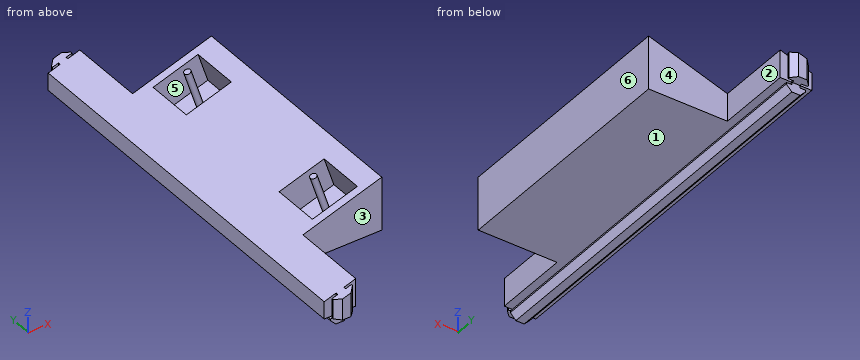
```python
from build123d import *

# Parameters (mm, degrees)
ESQUISSE1_W                   = 70
ESQUISSE1_H                   = 261.4
BOSS_EXTRU_1_DEPTH            = 40
ENL_V_MAT_EXTRU_1_DEPTH       = 335.841640665
ENL_V_MAT_EXTRU_1_DEPTH_BACK  = 40
ENL_V_MAT_EXTRU_2_DEPTH       = 335.841640665
ENL_V_MAT_EXTRU_2_DEPTH_BACK  = 40
ENL_V_MAT_EXTRU_3_DEPTH       = 287.347052656
ENL_V_MAT_EXTRU_3_DEPTH_BACK  = 165
ENL_V_MAT_EXTRU_4_DEPTH       = 328.480443637
ENL_V_MAT_EXTRU_4_DEPTH_BACK  = 261.4
ENL_V_MAT_EXTRU_5_DEPTH       = 328.480443637
ENL_V_MAT_EXTRU_5_DEPTH_BACK  = 261.4
ENL_V_MAT_EXTRU_6_DEPTH       = 335.841640665
ENL_V_MAT_EXTRU_6_DEPTH_BACK  = 40
ENL_V_MAT_EXTRU_8_DEPTH       = 335.841640665
ENL_V_MAT_EXTRU_8_DEPTH_BACK  = 40
ENL_V_MAT_EXTRU_9_DEPTH       = 281.544908808
ENL_V_MAT_EXTRU_9_DEPTH_BACK  = 40
ENL_V_MAT_EXTRU_10_DEPTH      = 335.841640665
ENL_V_MAT_EXTRU_10_DEPTH_BACK = 40
ENL_V_MAT_EXTRU_12_DEPTH      = 335.841640665
ENL_V_MAT_EXTRU_12_DEPTH_BACK = 40
ENL_V_MAT_EXTRU_14_DEPTH      = 280.494983601
ENL_V_MAT_EXTRU_14_DEPTH_BACK = 4.9
ENL_V_MAT_EXTRU_30_DEPTH      = 323.553128903
ENL_V_MAT_EXTRU_30_DEPTH_BACK = 323.553128903
ESQUISSE33_W                  = 30
ESQUISSE33_H                  = 30
ENL_V_MAT_EXTRU_34_DEPTH      = 20
ESQUISSE36_W                  = 30
ESQUISSE36_H                  = 30
ENL_V_MAT_EXTRU_35_DEPTH      = 20
ESQUISSE38_R                  = 2
BOSS_EXTRU_2_DEPTH            = 30
ESQUISSE39_R                  = 2
BOSS_EXTRU_3_DEPTH            = 30


with BuildPart() as part:
    # Esquisse1 → Boss.-Extru.1 (new body)
    with BuildSketch(Plane.XY):
        with Locations((-158.166976901, -139.865044598)):
            Rectangle(ESQUISSE1_W, ESQUISSE1_H)
    extrude(amount=BOSS_EXTRU_1_DEPTH)

    # Esquisse3 → Enlèv. mat.-Extru.1 (cut, two sides: drawn at the far end of the back side and taken through both)
    with BuildSketch(Plane.XY.offset(40).offset(-ENL_V_MAT_EXTRU_1_DEPTH_BACK)):
        Polygon((-173.166976901, 533.112927894), (-173.166976901, -9.165044598), (-173.166976901, -63.005044598), (-123.166976901, -63.005044598), (419.110995591, -63.005044598), (1188.481875045, 701.409795425), (596.203902553, 1297.527767917), align=None)
    extrude(amount=ENL_V_MAT_EXTRU_1_DEPTH + ENL_V_MAT_EXTRU_1_DEPTH_BACK, mode=Mode.SUBTRACT)

    # Esquisse4 → Enlèv. mat.-Extru.2 (cut, two sides: drawn at the far end of the back side and taken through both)
    with BuildSketch(Plane.XY.offset(40).offset(-ENL_V_MAT_EXTRU_2_DEPTH_BACK)):
        Polygon((-173.166976901, -812.84301709), (-173.166976901, -270.565044598), (-173.166976901, -216.725044598), (-123.166976901, -216.725044598), (419.110995591, -216.725044598), (1188.481875045, -981.139884621), (596.203902553, -1577.257857113), align=None)
    extrude(amount=ENL_V_MAT_EXTRU_2_DEPTH + ENL_V_MAT_EXTRU_2_DEPTH_BACK, mode=Mode.SUBTRACT)

    # Esquisse6 → Enlèv. mat.-Extru.3 (cut, two sides: drawn at the far end of the back side and taken through both)
    with BuildSketch(Plane(origin=(0, -63.005044598, 0), x_dir=(1, 0, 0), z_dir=(0, 1, 0)).offset(-ENL_V_MAT_EXTRU_3_DEPTH_BACK)):
        Polygon((42.299289537, -6.2), (-123.166976901, -6.2), (-173.166976901, -6.2), (-173.166976901, 0), (-173.166976901, 165.466266437), (33.046852916, 424.294776666), (248.513119354, 252.628510228), align=None)
    extrude(amount=ENL_V_MAT_EXTRU_3_DEPTH + ENL_V_MAT_EXTRU_3_DEPTH_BACK, mode=Mode.SUBTRACT)

    # Esquisse7 → Enlèv. mat.-Extru.4 (cut, two sides: drawn at the far end of the back side and taken through both)
    with BuildSketch(Plane(origin=(0, -9.165044598, 0), x_dir=(1, 0, 0), z_dir=(0, 1, 0)).offset(-ENL_V_MAT_EXTRU_4_DEPTH_BACK)):
        Polygon((-23.31660268, -6.2), (-173.166976901, -6.2), (-180.716976901, -6.2), (-180.716976901, -4.65), (-177.016976901, -4.65), (-177.016976901, -3.65), (-180.521416942, 0), (-284.304352032, 108.093649388), (-164.080204276, 382.623598415), (96.907545076, 268.329949026), align=None)
    extrude(amount=ENL_V_MAT_EXTRU_4_DEPTH + ENL_V_MAT_EXTRU_4_DEPTH_BACK, mode=Mode.SUBTRACT)

    # Esquisse8 → Enlèv. mat.-Extru.5 (cut, two sides: drawn at the far end of the back side and taken through both)
    with BuildSketch(Plane(origin=(0, -9.165044598, 0), x_dir=(1, 0, 0), z_dir=(0, 1, 0)).offset(-ENL_V_MAT_EXTRU_5_DEPTH_BACK)):
        Polygon((-358.633243338, -6.2), (-193.166976901, -6.2), (-185.616976901, -6.2), (-185.616976901, -4.65), (-189.316976901, -4.65), (-189.316976901, -3.65), (-185.81253686, 0), (-71.214392687, 119.358077569), (-203.692164198, 422.617012095), (-491.11101485, 297.058934527), align=None)
    extrude(amount=ENL_V_MAT_EXTRU_5_DEPTH + ENL_V_MAT_EXTRU_5_DEPTH_BACK, mode=Mode.SUBTRACT)

    # Esquisse9 → Enlèv. mat.-Extru.6 (cut, two sides: drawn at the far end of the back side and taken through both)
    with BuildSketch(Plane.XY.offset(40).offset(-ENL_V_MAT_EXTRU_6_DEPTH_BACK)):
        Polygon((-740.770645722, -15.365044598), (-193.166976901, -15.365044598), (-185.616976901, -15.365044598), (-185.616976901, -13.815044598), (-189.316976901, -13.815044598), (-189.316976901, -12.815044598), (-185.81253686, -9.165044598), (193.445214828, 385.845507022), (-238.735419917, 1392.174981587), (-1172.951280468, 990.964429967), align=None)
    extrude(amount=ENL_V_MAT_EXTRU_6_DEPTH + ENL_V_MAT_EXTRU_6_DEPTH_BACK, mode=Mode.SUBTRACT)

    # Esquisse10 → Enlèv. mat.-Extru.8 (cut, two sides: drawn at the far end of the back side and taken through both)
    with BuildSketch(Plane.XY.offset(40).offset(-ENL_V_MAT_EXTRU_8_DEPTH_BACK)):
        Polygon((372.069388801, -15.365044598), (-173.166976901, -15.365044598), (-180.716976901, -15.365044598), (-180.716976901, -13.815044598), (-177.016976901, -13.815044598), (-177.016976901, -12.815044598), (-180.521416942, -9.165044598), (-558.13962874, 384.13786742), (-127.815363107, 1386.111821344), (802.393654434, 986.608909326), align=None)
    extrude(amount=ENL_V_MAT_EXTRU_8_DEPTH + ENL_V_MAT_EXTRU_8_DEPTH_BACK, mode=Mode.SUBTRACT)

    # Esquisse11 → Enlèv. mat.-Extru.9 (cut, two sides: drawn at the far end of the back side and taken through both)
    with BuildSketch(Plane.ZY.offset(185.616976901).offset(-ENL_V_MAT_EXTRU_9_DEPTH_BACK)):
        Polygon((-537.152349895, -15.365044598), (0, -15.365044598), (6.2, -15.365044598), (6.2, -9.165044598), (6.2, 527.987305297), (-753.448138282, 1287.635443579), (-1296.800488177, 744.283093684), align=None)
    extrude(amount=ENL_V_MAT_EXTRU_9_DEPTH + ENL_V_MAT_EXTRU_9_DEPTH_BACK, mode=Mode.SUBTRACT)

    # Esquisse12 → Enlèv. mat.-Extru.10 (cut, two sides: drawn at the far end of the back side and taken through both)
    with BuildSketch(Plane.XY.offset(40).offset(-ENL_V_MAT_EXTRU_10_DEPTH_BACK)):
        Polygon((372.069388801, -264.365044598), (-173.166976901, -264.365044598), (-180.716976901, -264.365044598), (-180.716976901, -265.915044598), (-177.016976901, -265.915044598), (-177.016976901, -266.915044598), (-180.521416942, -270.565044598), (-558.13962874, -663.867956616), (-127.815363107, -1665.84191054), (802.393654434, -1266.338998522), align=None)
    extrude(amount=ENL_V_MAT_EXTRU_10_DEPTH + ENL_V_MAT_EXTRU_10_DEPTH_BACK, mode=Mode.SUBTRACT)

    # Esquisse13 → Enlèv. mat.-Extru.12 (cut, two sides: drawn at the far end of the back side and taken through both)
    with BuildSketch(Plane.XY.offset(40).offset(-ENL_V_MAT_EXTRU_12_DEPTH_BACK)):
        Polygon((-740.770645722, -264.365044598), (-193.166976901, -264.365044598), (-185.616976901, -264.365044598), (-185.616976901, -265.915044598), (-189.316976901, -265.915044598), (-189.316976901, -266.915044598), (-185.81253686, -270.565044598), (193.445214828, -665.575596218), (-238.735419917, -1671.905070783), (-1172.951280468, -1270.694519163), align=None)
    extrude(amount=ENL_V_MAT_EXTRU_12_DEPTH + ENL_V_MAT_EXTRU_12_DEPTH_BACK, mode=Mode.SUBTRACT)

    # Esquisse16 → Enlèv. mat.-Extru.14 (cut, two sides: drawn at the far end of the back side and taken through both)
    with BuildSketch(Plane(origin=(-180.716976901, 0, 0), x_dir=(0, 0, -1), z_dir=(1, 0, 0)).offset(-ENL_V_MAT_EXTRU_14_DEPTH_BACK)):
        Polygon((537.152349895, -264.365044598), (0, -264.365044598), (-6.2, -264.365044598), (-6.2, -270.565044598), (-6.2, -807.717394493), (753.448138282, -1567.365532776), (1296.800488177, -1024.01318288), align=None)
    extrude(amount=ENL_V_MAT_EXTRU_14_DEPTH + ENL_V_MAT_EXTRU_14_DEPTH_BACK, mode=Mode.SUBTRACT)


with BuildPart() as enl_v_mat_extru_14_kept_piece:
    # of the separate pieces the step leaves, the one the design keeps (enl_v_mat_extru_14_pieces_kept)
    add(part.part.solids().sort_by_distance((-193.166976901, -264.365044598, 6.2))[0])

    # Esquisse32 → Enlèv. mat.-Extru.30 (cut, two sides: drawn at the far end of the back side and taken through both)
    with BuildSketch(Plane(origin=(0, -264.365044598, 0), x_dir=(-1, 0, 0), z_dir=(0, -1, 0)).offset(-ENL_V_MAT_EXTRU_30_DEPTH_BACK)):
        Polygon((364.412131867, -40), (193.166976901, -40), (123.166976901, -40), (193.166976901, -17.255621264), (356.030797415, 35.662041825), (696.438947848, 73.370177768), (704.8202823, -2.291864057), align=None)
    extrude(amount=ENL_V_MAT_EXTRU_30_DEPTH + ENL_V_MAT_EXTRU_30_DEPTH_BACK, mode=Mode.SUBTRACT)

    # Esquisse33 → Enlèv. mat.-Extru.34 (cut)
    with BuildSketch(Plane(origin=(-23.517104767, 0, 72.378206183), x_dir=(0.9510565162951555, 0, 0.3090169943749416), z_dir=(-0.3090169943749416, 0, 0.9510565162951555))):
        with Locations((-132.351187411, -83.005044598)):
            Rectangle(ESQUISSE33_W, ESQUISSE33_H)
    extrude(amount=-ENL_V_MAT_EXTRU_34_DEPTH, mode=Mode.SUBTRACT)

    # Esquisse36 → Enlèv. mat.-Extru.35 (cut)
    with BuildSketch(Plane(origin=(-23.517104767, 0, 72.378206183), x_dir=(0.9510565162951555, 0, 0.3090169943749416), z_dir=(-0.3090169943749416, 0, 0.9510565162951555))):
        with Locations((-132.351187411, -196.725044598)):
            Rectangle(ESQUISSE36_W, ESQUISSE36_H)
    extrude(amount=-ENL_V_MAT_EXTRU_35_DEPTH, mode=Mode.SUBTRACT)

    # Esquisse38 → Boss.-Extru.2 (add)
    with BuildSketch(Plane(origin=(-17.336764879, 0, 53.357075857), x_dir=(0.9510565162951555, 0, 0.3090169943749415), z_dir=(-0.3090169943749415, 0, 0.9510565162951556))):
        with Locations((-132.351187411, -83.005044598)):
            Circle(ESQUISSE38_R)
    extrude(amount=BOSS_EXTRU_2_DEPTH)

    # Esquisse39 → Boss.-Extru.3 (add)
    with BuildSketch(Plane(origin=(-17.336764879, 0, 53.357075857), x_dir=(0.9510565162951555, 0, 0.3090169943749415), z_dir=(-0.3090169943749415, 0, 0.9510565162951556))):
        with Locations((-132.351187411, -196.725044598)):
            Circle(ESQUISSE39_R)
    extrude(amount=BOSS_EXTRU_3_DEPTH)


solid = enl_v_mat_extru_14_kept_piece.part
```
Can you work these out from the model? Positions are in its coordinate system, mm. Face numbers are marked on the shaded views. A direction names the side the tool comes from. Round coordinates to 2 decimals unless told otherwise and drop trailing zeros. Loops run counter-clockwise (first coordinate to the right, second up) from the corner with the lowest first, then second, coordinate; pieces in that order, holes last. Notation, with made-up numbers: M 35,22.25 L 68,22.25 A29 cw 68,50.25 Z; hole C 35.5,35.25 d10. An arc over 180 degrees is marked long. Write item = value, one per line. Start each with the question number.
(1) I'm going to push flat-ended pins straight in: P1, Ø3, axis at x = -148, z = 20, coming from the -Y side; P2, Ø0.5, axis at y = -266.5, z = 16.5, coming from the +X side; P3, Ø0.8, axis at y = -163.5, z = 4.5, coming from the -X side. Where does each tip first touch, or does it pass through?
(2) I need wall thicknesses on line 1 along Y through (x, z) = (-144.5, 25.5); line 2 along Z through (x, y) = (-185.5, -107.5); line 3 along Y through (x, z) = (-151.5, 9.5). Which ranges of each line are inside material? Lowest first, please.
(3) Which directions (+Z, -Z, +X, -X, +Y, -Y) give clear straight access to the entire face, cutting with the end or side of a thin tool? Please do the marked faces 1, 2 and 3.
(4) Suppose I cut it at A-A on y = -172. Write out the boundary of the cut face in (x, z).
(5) If we mould it in two halves opening along X, with no side actions, what happens to the marked faces 4, 5 and 6? For each: released by +X, released by -X, zero draft, split by the parting line, or undercut.
(6) Suppose I cut it at B-B on z = 30.5. Give the number of separate pieces and of enclosed holes in the cut face, plus the area to 3 significant figures.
(7) Suppose I cut it at C-C on y = -230. Write out the boundary of the cut face in (x, z).
Answer block:
q1.P1 = -216.73
q1.P2 = -177.02
q1.P3 = -189.32
q2.line_1 = -216.73 to -211.73, -181.73 to -98.01, -68.01 to -63.01
q2.line_2 = 0 to 19.75
q2.line_3 = -216.73 to -63.01
q3.face_1 = +X, +Y, -Y
q3.face_2 = +Z, -Z, +X, +Y
q3.face_3 = +Z, -Z, +X, -Y
q4.outline = M -193.17,6.2 L -185.62,6.2 L -185.62,4.65 L -189.32,4.65 L -189.32,3.65 L -185.81,0 L -180.52,0 L -177.02,3.65 L -177.02,4.65 L -180.72,4.65 L -180.72,6.2 L -123.17,6.2 L -123.17,40 L -193.17,17.26 Z
q5.face_4 = zero draft
q5.face_5 = undercut
q5.face_6 = released by +X
q6.separate_pieces = 3
q6.enclosed_holes = 0
q6.area = 3,370 mm²
q7.outline = M -193.17,6.2 L -185.62,6.2 L -185.62,4.65 L -189.32,4.65 L -189.32,3.65 L -185.81,0 L -180.52,0 L -177.02,3.65 L -177.02,4.65 L -180.72,4.65 L -180.72,6.2 L -173.17,6.2 L -173.17,23.75 L -193.17,17.26 Z
